Part print with two shaded views. Sizes in mm from the minimum x, y, z corner. Round coordinates to 2 decimals unless told otherwise and drop trailing zeros. Write each loop counter-clockwise with the first axis right and the second up, starting at its lowest first coordinate (ties: lowest second). Pieces come first, ordered by that corner, then holes. Notation, with made-up numbers: (41, -30.75) - (45, -30.75) arc R10 cw to (45, -25.75) - close; hole circle Ø7 at (39.5, 80). An arc over 180 degrees is marked (long way). Answer as a JSON object with one key per item and string values. Group by question number.
Item 1: Slice it at C-C, the plane x = 3.5. List the corners of the cut face in (y, z) (1 decimal).
Item 2: Slice it at B-B, the plane z = 7. List the corners of the cut face in (x, y) (1 decimal).
Item 3: Flat gauge pin, fed straight in: pin 1 (2.5 mm diameter, centred on x = 38.29, z = 6.35, fed in from -Y). Where does the tip first touch, or does it go through?
Item 4: Probe line 1 (Z direction, x = 6, y = 0.4) (1 decimal); line 2 (Z direction, x = 37.5, y = 0.6) (1 decimal); line 3 (X direction, y = 0.45, z = 20.75) (1 decimal). List the from-to ranges inside material, lowest first. Write a range as from..to.
Item 5: Slice it at A-A, the plane y = 0.7. Give the number of separate pieces and of enclosed holes in the cut face, then the cut area to 3 significant figures.
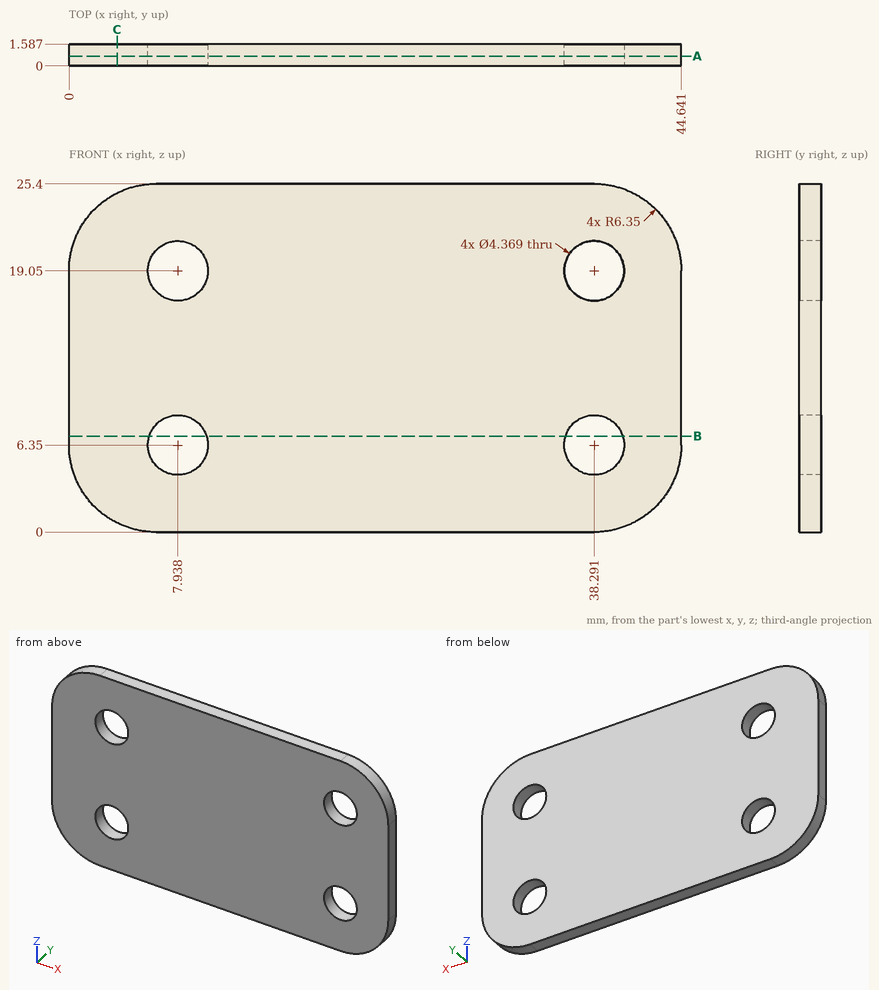
Geometry says:
{
 "1": {"outline": "(0, 0.7) - (1.6, 0.7) - (1.6, 24.7) - (0, 24.7) - close"},
 "2": {"outline": "(0, 0) - (5.9, 0) - (5.9, 1.6) - (0, 1.6) - close; (10, 0) - (36.2, 0) - (36.2, 1.6) - (10, 1.6) - close; (40.4, 0) - (44.6, 0) - (44.6, 1.6) - (40.4, 1.6) - close"},
 "3": {"pin 1": "passes through"},
 "4": {"line 1": "z = 0..5.3, 7.4..18, 20.1..25.4", "line 2": "z = 0..4.3, 8.4..17, 21.1..25.4", "line 3": "x = 0.2..6.6, 9.3..36.9, 39.7..44.4"},
 "5": {"separate pieces": "1", "enclosed holes": "4", "area": "1,040 mm^2"}
}
